Geometry: final body of the model. Coordinates: model frame, mm. A direction names the side the tool comes from. Coordinates: 2 decimals unless noted, no trailing zeros. Write each loop counter-clockwise with the first axis right and the second up, starting at its lowest first coordinate (ties: lowest second). Pieces come first, ordered by that corner, then holes. Notation, with made-up numbers: M 61,77.25 L 96,77.25 A34 ccw 96,111.25 Z; hole C -29.5,-18.5 d1. An arc over 180 degrees is marked long. Write item = value, one per line. Start each with the question number.
Item 1: Section A-A on y = 0. Output: boundary loops of the cut face in (x, z).
Item 2: Pull-direction query (Y, two-part tool) for faces 4 (the cylindrical face through (25.845, -22.858, -2.348)), 5 (the flat face through (28.178, 0, -2)), 6 (the cylindrical face through (3.64, -27.7, -26.68)); classes: +Y half, -Y half, draft (parallel to the pull), parting line (faces both ways), or undercut.
Item 3: Section D-D on x = 15. Output: boundary loops of the cut face in (y, z).
Item 4: Ray query, L1, parallel to Z at x = -24, y = -13; L2, parallel to Z at x = -20, y = -26; L3, parallel to Y at x = -0.5, z = -40.5. Return the intervals inside material, ascending. Write a range as [from, to].
Item 5: First-contact query: pin 1 Ø4.5 at (x, y) = (0, 0) entering from -Z; pin 2 Ø1.5 at (x, y) = (-21, 7.5) entering from +Z; pin 3 Ø5.5 at (x, y) = (23.57, -23.57) entering from -Z; pin 4 Ø4 at (y, z) = (-0.5, -33) entering from -X. Flat tips, straight axial feed; report the tip coordinate or a pass-through.
Item 6: Section C-C on z = -31.5. Output: boundary loops of the cut face in (x, y), plus the area to 3 significant figures.
Item 7: Reachability of faces 1 (the flat face through (-28.178, 0, -2)), 2 (the flat face through (-0.4, 19.2, 0)), 3 (the flat face through (-25, 13, -4.762)) from +Z, -Z, +X, -X, +Y, -Y: full face, straight path, thin tool, end or side. Return the list, or none.
Autodesk Inventor part; units mm, degrees
ref_plane "YZ Plane" through (0, 0, 0) normal (1, 0, 0) x (0, 1, 0)
ref_plane "XZ Plane" through (0, 0, 0) normal (0, 1, 0) x (-1, 0, 0)
ref_plane "XY Plane" through (0, 0, 0) normal (0, 0, 1) x (1, 0, 0)
sketch "Sketch1" plane through (0, 0, 0) normal (0, 0, 1) x (1, 0, 0)
  line L0 (-28.1781, -28.1781) -> (28.1781, -28.1781)
  line L1 (28.1781, -28.1781) -> (28.1781, 28.1781)
  line L2 (28.1781, 28.1781) -> (-28.1781, 28.1781)
  line L3 (-28.1781, 28.1781) -> (-28.1781, -28.1781)
  line L4 (-28.1781, -28.1781) -> (28.1781, 28.1781) construction
  line L5 (28.1781, -28.1781) -> (-28.1781, 28.1781) construction
  circle A0 centre (-23.5732, 23.5732) radius 2.3813
  circle A1 centre (23.5732, 23.5732) radius 2.3813
  circle A2 centre (23.5732, -23.5732) radius 2.3813
  circle A3 centre (-23.5732, -23.5732) radius 2.3813
  circle A4 centre (0, 0) radius 3.556
  dimension "d0" = 56.3563
  dimension "d1" = 56.3563
extrude "Extrusion1" add sketch "Sketch1" against normal blind 4.7625
sketch "Sketch2" plane through (0, 0, 0) normal (0, 0, 1) x (1, 0, 0)
  circle A0 centre (0, 0) radius 3.556
  circle A1 centre (0, 0) radius 3.556
  circle A2 centre (0, 0) radius 19.05
  dimension "d4" = 38.1
extrude "Extrusion2" add sketch "Sketch2" along normal blind 0.7937
sketch "Sketch3" plane through (0, 0, -4.7625) normal (0, 0, -1) x (-1, 0, 0)
  circle A0 centre (0, 0) radius 3.556
  circle A1 centre (0, 0) radius 27.94
  dimension "d7" = 55.88
extrude "Extrusion3" add sketch "Sketch3" along normal blind 44.45
properties part number "stepperMotorBody" material "Steel, Galvanized"
Responses:
q1.outline = M -28.18,-4.76 L -27.94,-4.76 L -27.94,-49.21 L -3.56,-49.21 L -3.56,0.79 L -19.05,0.79 L -19.05,0 L -28.18,0 Z; M 3.56,-49.21 L 27.94,-49.21 L 27.94,-4.76 L 28.18,-4.76 L 28.18,0 L 19.05,0 L 19.05,0.79 L 3.56,0.79 Z
q2.face_4 = undercut
q2.face_5 = draft
q2.face_6 = parting line
q3.outline = M -28.18,-4.76 L -23.57,-4.76 L -23.57,-49.21 L 23.57,-49.21 L 23.57,-4.76 L 28.18,-4.76 L 28.18,0 L 11.74,0 L 11.74,0.79 L -11.74,0.79 L -11.74,0 L -28.18,0 Z
q4.L1 = [-49.21, 0]
q4.L2 = [-4.76, 0]
q4.L3 = [-27.94, -3.52], [3.52, 27.94]
q5.pin_1 = through
q5.pin_2 = 0
q5.pin_3 = -4.76
q5.pin_4 = -27.94
q6.outline = C 0,0 d55.88; hole C 0,0 d7.11
q6.area = 2,410 mm²
q7.face_1 = +Z, -Z, -X, +Y, -Y
q7.face_2 = +Z
q7.face_3 = -Z
